Here's how the part is built. I have some questions about the finished solid (model axes, mm). Coordinates: 2 decimals unless noted, no trailing zeros. Write each loop counter-clockwise with the first axis right and the second up, starting at its lowest first coordinate (ties: lowest second). Pieces come first, ordered by that corner, then holes. Notation, with made-up numbers: M 16,5.5 L 29,5.5 A8 cw 29,20.5 Z; hole C -26.5,-31.75 d6. An arc over 180 degrees is marked long. Write each question's results on one line, items separated by ' | '. Start each with the question number.
from build123d import *

# Parameters (mm, degrees)
SKETCH3_R           = 3
BOSS_EXTRUDE2_DEPTH = 1.75


with BuildPart() as part:
    # Sketch3 → Boss-Extrude2 (new, symmetric)
    with BuildSketch(Plane(origin=(0, 0, 0), x_dir=(0, 0, -1), z_dir=(1, 0, 0))):
        with BuildLine():
            Line((3, 0), (12, 0))
            ThreePointArc((12, 0), (14.121320344, -0.878679656), (15, -3))
            Line((15, -3), (15, -67))
            ThreePointArc((15, -67), (14.121320344, -69.121320344), (12, -70))
            Line((12, -70), (3, -70))
            ThreePointArc((3, -70), (0.878679656, -69.121320344), (0, -67))
            Line((0, -67), (0, -3))
            ThreePointArc((0, -3), (0.878679656, -0.878679656), (3, 0))
        make_face()
        with Locations((7.5, -5)):
            Circle(SKETCH3_R, mode=Mode.SUBTRACT)
        with Locations((7.5, -65)):
            Circle(SKETCH3_R, mode=Mode.SUBTRACT)
    extrude(amount=BOSS_EXTRUDE2_DEPTH, both=True)


solid = part.part
1) I want a section at C-C, the plane z = -7.5. Write out the boundary of the cut face in (x, y).
2) We'd pull the mould along Y, two halves only. Please class faces 1 (the cylindrical face through (0.02, -0.86, -14.1)), 2 (the flat face through (0, -35, 0)), 3 (the cylindrical face through (-0.024, -67.662, -8.884)): pulls with the +Y half, pulls with the -Y half, needs draft (parallel to the pull), parting line crosses it, or undercut.
3) For pin 1 Ø3.5 at (y, z) = (-65, -7.5) entering from +X, with a flat end and sliding along its axis, tell me the tip position at first contact or that it passes through.
4) Please list where these lines run through material, in increasing order: line 1 (Y direction, x = -0.5, z = -7.5); line 2 (Y direction, x = 1.25, z = -4.75); line 3 (Z direction, x = 0.5, y = -63.5). Write a range as [from, to].
5) I want a section at A-A, the plane x = 0.05. Write out the boundary of the cut face in (y, z), then the cut area to 3 significant figures.
6) I want a section at B-B, the plane y = -65. Write out the boundary of the cut face in (x, z), then the cut area to 3 significant figures.
Output:
1) outline: M -1.75,-70 L 1.75,-70 L 1.75,-68 L -1.75,-68 Z; M -1.75,-62 L 1.75,-62 L 1.75,-8 L -1.75,-8 Z; M -1.75,-2 L 1.75,-2 L 1.75,0 L -1.75,0 Z
2) face 1: pulls with the +Y half | face 2: needs draft | face 3: undercut
3) pin 1: passes through
4) line 1: y = [-70, -68], [-62, -8], [-2, 0] | line 2: y = [-70, -66.2], [-63.8, -6.2], [-3.8, 0] | line 3: z = [-15, -10.1], [-4.9, 0]
5) outline: M -70,-12 A3 ccw -67,-15 L -3,-15 A3 ccw 0,-12 L 0,-3 A3 ccw -3,0 L -67,0 A3 ccw -70,-3 Z; hole C -65,-7.5 d6; hole C -5,-7.5 d6 | area: 986 mm2
6) outline: M -1.75,-15 L 1.75,-15 L 1.75,-10.5 L -1.75,-10.5 Z; M -1.75,-4.5 L 1.75,-4.5 L 1.75,0 L -1.75,0 Z | area: 31.5 mm2
